Input: part model. Units: mm. Frame: model coordinates. A direction names the side the tool comes from. Coordinates: 2 decimals unless noted, no trailing zeros. Order: outer loops, then holes, each group sorted by start corner. A loop starts at its lowest first (then second) coordinate and runs counter-clockwise, first axis right, second up. Notation, with made-up numbers: (-18.5, 28.5) -> (28.5, 28.5) arc R20 cw to (28.5, 35.5) -> close; hole circle Ø2 at (-29, 61.5). An arc over 180 degrees is marked (long way). One line per item, written item: value. Start each with the question number.
from build123d import *

# Parameters (mm, degrees)
ESQUISSE1_W             = 23
ESQUISSE1_H             = 4
ESQUISSE2_W             = 20
ESQUISSE2_H             = 10
ENL_V_MAT_EXTRU_1_DEPTH = 0.5
CHANFREIN1_SIZE         = 0.5


with BuildPart() as part:
    # Esquisse1 → Révolution1 (revolve)
    with BuildSketch(Plane.XY, mode=Mode.PRIVATE) as r_volution1_sk:
        with Locations((11.5, 2)):
            Rectangle(ESQUISSE1_W, ESQUISSE1_H)
    revolve(r_volution1_sk.sketch.rotate(Axis((-20.595505618, 0, 0), (1, 0, 0)), 90), axis=Axis((-20.595505618, 0, 0), (1, 0, 0)))

    # Esquisse2 → Enlèv. mat.-Extru.1 (cut)
    with BuildSketch(Plane.XY.offset(4)):
        with Locations((10, 0)):
            Rectangle(ESQUISSE2_W, ESQUISSE2_H)
    extrude(amount=-ENL_V_MAT_EXTRU_1_DEPTH, mode=Mode.SUBTRACT)

    # Chanfrein1
    chanfrein1_edges = [part.edges().sort_by_distance(p)[0] for p in [
        (0, 0, -4),
    ]]
    chamfer(chanfrein1_edges, length=CHANFREIN1_SIZE - 0.0001)  # a hair under: the kernel refuses the full size


solid = part.part
1) Section query A-A, the plane x = 14.5. Return the cut outline in (y, z).
2) Pin query (flat end, axial travel): pin 1 Ø3 at (x, y) = (4.5, 2.5) entering from -Z; pin 2 Ø1.2 at (x, y) = (6, 0) entering from +Z; pin 3 Ø4 at (x, z) = (12.5, -3) entering from -Y; pin 4 Ø2 at (x, y) = (19.5, -0.5) entering from -Z. Return the tip coordinate at first contact, or that it passes through.
3) Ray query, line 1 along Z through (x, y) = (6, -3.5); line 2 along Z through (x, y) = (12, 0). Return the intervals inside material, ascending. Write a range as from..to.
4) Access query for faces 1 (the conical face through (0.142, -0.16, -3.639)), 2 (the flat face through (10, 0, 3.5)). Directions: +Z, -Z, +X, -X, +Y, -Y. A direction counts if a zero-diameter tool reaches every point of the face in a straight line with its end or side. Return the directions, or none.
Entries:
1. outline: (-1.94, 3.5) arc R4 ccw (long way) to (1.94, 3.5) -> close
2. pin 1: stops at z = -3.87
2. pin 2: stops at z = 3.5
2. pin 3: stops at y = -3.87
2. pin 4: stops at z = -4
3. line 1: z = -1.94..1.94
3. line 2: z = -4..3.5
4. face 1: -X
4. face 2: +Z, -X, +Y, -Y
